```python
from build123d import *

# Parameters (mm, degrees)
F1_DEPTH  = 14
F2_W      = 3
F2_H      = 11.408352
F3_DEPTH  = 18
F5_DEPTH  = 25
F6_R      = 2.8
F7_DEPTH  = 25
F8_R      = 5.75
F9_DEPTH  = 1.5
F10_W     = 3
F10_H     = 9.991856
F11_DEPTH = 18
F13_DEPTH = 25
F14_R     = 2.8
F15_DEPTH = 25
F16_R     = 5.75
F17_DEPTH = 1.5


with BuildPart() as f1:
    # F0 (on Top) → F1 (new body)
    with BuildSketch(Plane.XY):
        with BuildLine():
            Line((-5.879243, 26.052212), (-25.879243, 26.052212))
            Line((-25.879243, 26.052212), (-25.879243, 11.060356))
            ThreePointArc((-25.879243, 11.060356), (-24.293036, 0.175264), (-19.988959, -9.947788))
            ThreePointArc((-19.988959, -9.947788), (-18.281685, -12.624792), (-16.380951, -15.168086))
            ThreePointArc((-16.380951, -15.168086), (-2.161149, -18.102259), (0, -3.744627))
            ThreePointArc((0, -3.744627), (-0.595324, -3.130936), (-1.163612, -2.492127))
            ThreePointArc((-1.163612, -2.492127), (-4.546963, 3.177378), (-5.879243, 9.64386))
            ThreePointArc((-5.879243, 9.64386), (-5.891908, 10.352108), (-5.879243, 11.060356))
            Line((-5.879243, 11.060356), (-5.879243, 26.052212))
        make_face()
        with BuildLine():
            ThreePointArc((-3.681243, -9.899788), (-7.857243, -14.099719), (-12.080969, -9.947788))
            ThreePointArc((-12.080969, -9.947788), (-10.050272, -6.303218), (-5.879243, -6.207635))
            ThreePointArc((-5.879243, -6.207635), (-4.272338, -7.751347), (-3.681243, -9.899788))
        make_face(mode=Mode.SUBTRACT)
        with BuildLine():
            Line((-5.879243, 9.64386), (-5.879243, 11.060356))
            ThreePointArc((-5.879243, 11.060356), (-5.891908, 10.352108), (-5.879243, 9.64386))
        make_face()
        with BuildLine():
            ThreePointArc((0, -3.744627), (-0.554991, -3.093465), (-1.163612, -2.492127))
            ThreePointArc((-1.163612, -2.492127), (-0.595324, -3.130936), (0, -3.744627))
        make_face()
    extrude(amount=F1_DEPTH)

    # F2 (on face) → F3 (join)
    with BuildSketch(Plane.XY.offset(14)):
        Polygon((-5.879243, 26.052212), (-25.879243, 26.052212), (-25.879243, 21.052212), (-22.879243, 21.052212), (-8.879243, 21.052212), (-5.879243, 21.052212), align=None)
        with BuildLine():
            Line((-22.879243, 21.052212), (-25.879243, 21.052212))
            Line((-25.879243, 21.052212), (-25.879243, 11.060356))
            ThreePointArc((-25.879243, 11.060356), (-25.862016, 10.351917), (-25.83308, 9.64386))
            Line((-25.83308, 9.64386), (-22.879243, 9.64386))
            Line((-22.879243, 9.64386), (-22.879243, 21.052212))
        make_face()
        with Locations((-7.379243, 15.348036)):
            Rectangle(F2_W, F2_H)
    extrude(amount=F3_DEPTH)

    # F4 (on face) → F5 (cut)
    with BuildSketch(Plane.YZ.offset(-5.879243)):
        Polygon((9.64386, 14), (23.052212, 32), (9.64386, 32), align=None)
    extrude(amount=-F5_DEPTH, mode=Mode.SUBTRACT)

    # F6 (on face) → F7 (cut)
    with BuildSketch(Plane.XZ.offset(-21.052212)):
        with Locations((-15.879243, 21.657553)):
            Circle(F6_R)
    extrude(amount=-F7_DEPTH, mode=Mode.SUBTRACT)

    # F8 (on face) → F9 (cut)
    with BuildSketch(Plane.XZ.offset(-21.052212)):
        with Locations((-15.879243, 21.657553)):
            Circle(F8_R)
    extrude(amount=-F9_DEPTH, mode=Mode.SUBTRACT)

    # F10 (on face) → F11 (join)
    with BuildSketch(Plane(origin=(0, 0, 0), x_dir=(1, 0, 0), z_dir=(0, 0, -1))):
        with Locations((-24.379243, -16.056284)):
            Rectangle(F10_W, F10_H)
        Polygon((-25.879243, -21.052212), (-25.879243, -26.052212), (-5.879243, -26.052212), (-5.879243, -21.052212), (-8.879243, -21.052212), (-22.879243, -21.052212), align=None)
        with Locations((-7.379243, -16.056284)):
            Rectangle(F10_W, F10_H)
    extrude(amount=F11_DEPTH)

    # F12 (on face) → F13 (cut)
    with BuildSketch(Plane(origin=(-25.879243, 0, 0), x_dir=(0, -1, 0), z_dir=(-1, 0, 0))):
        Polygon((-11.060356, 0), (-22.052212, -18), (-11.060356, -18), align=None)
    extrude(amount=-F13_DEPTH, mode=Mode.SUBTRACT)

    # F14 (on face) → F15 (cut)
    with BuildSketch(Plane.XZ.offset(-21.052212)):
        with Locations((-15.879243, -8.181212)):
            Circle(F14_R)
    extrude(amount=-F15_DEPTH, mode=Mode.SUBTRACT)

    # F16 (on face) → F17 (cut)
    with BuildSketch(Plane.XZ.offset(-21.052212)):
        with Locations((-15.879243, -8.181212)):
            Circle(F16_R)
    extrude(amount=-F17_DEPTH, mode=Mode.SUBTRACT)


solid = f1.part
```
The model under review builds one solid part; all positions refer to its coordinate system, in mm. A direction names the side the tool comes from. Round coordinates to 2 decimals unless told otherwise and drop trailing zeros. Write each loop counter-clockwise with the first axis right and the second up, starting at its lowest first coordinate (ties: lowest second). Pieces come first, ordered by that corner, then holes. Notation, with made-up numbers: (-19.5, 42) - (29.5, 42) arc R32 ccw to (29.5, 78) - close; hole circle Ø1 at (64, 83). An arc over 180 degrees is marked (long way). One line per question, with ' | ' between items.
Item 1: Add section B-B, the plane x = -18. Give the boundary of the cut face in (y, z).
Resolved:
outline: (-13.03, 0) - (21.05, 0) - (21.05, -2.84) - (22.55, -2.84) - (22.55, -6.35) - (26.05, -6.35) - (26.05, 19.83) - (22.55, 19.83) - (22.55, 16.31) - (21.05, 16.31) - (21.05, 14) - (-13.03, 14) - close; (21.05, -16.36) - (22.05, -18) - (26.05, -18) - (26.05, -10.01) - (22.55, -10.01) - (22.55, -13.53) - (21.05, -13.53) - close; (21.05, 27) - (22.55, 27) - (22.55, 23.49) - (26.05, 23.49) - (26.05, 32) - (23.05, 32) - (21.05, 29.32) - close
Item 2: Add section C-C, the plane x = -7.25. Give the boundary of the cut face in (y, z).
Resolved:
outline: (-19.88, 0) - (-14.05, 0) - (-14.05, 14) - (-19.88, 14) - close; (-5.75, 0) - (11.06, 0) - (22.05, -18) - (26.05, -18) - (26.05, 32) - (23.05, 32) - (9.64, 14) - (-5.75, 14) - close
Item 3: For faces 1 (the face through (-5.879, 20, 7)), 2 (the face through (-8.879, 17, -6)), 3 (the face through (-10.568, 21.792, 19.455)), 4 (the face through (-12, 1, 14)), 5 (the face through (-13.21, 24.28, -7.34)), list the 3-axis set-ups (+Z, -Z, +X, -X, +Y, -Y) from which the entire face can be reached by the end or side of a thin tool; tool diameter is ignored.
Resolved:
face 1: +Z, -Z, +X, +Y | face 2: -Z, -Y | face 3: -Y | face 4: +Z, -Y | face 5: +Y, -Y
Item 4: The part is to be moulded in two halves that separate along X. For faces 6 (the face through (-4.513, 3.091, 6.902)), 7 (the face through (-25.879, 20, 7)), 8 (the face through (-2.35, -18.23, 6.9)), 9 (the face through (-13.21, 24.28, 22.5)), say which applies: pulls with the +X half, pulls with the -X half, needs draft (parallel to the pull), parting line crosses it, or undercut.
Resolved:
face 6: pulls with the +X half | face 7: pulls with the -X half | face 8: parting line crosses it | face 9: undercut
Item 5: For P1, Ø4, axis at x = -7, y = -11.5, coming from the +Z side; P2, Ø8, axis at y = 21.5, z = 7, coming from the +X side; P3, Ø8.5, axis at x = -9, y = 8.5, coming from the +Z side; P4, Ø4, axis at x = -15, z = 19, coming from the -Y side, all flat-tipped, find the tip position at first contact; note any pin that passes through.
Resolved:
P1: passes through | P2: stops at x = -5.88 | P3: stops at z = 18.17 | P4: stops at y = 22.55
Item 6: To check wall thickness, follow probe 1 along X at (y, z) = (19, 22.5); probe 2 along X at (y, z) = (15, 7.5); probe 3 along Z at (x, y) = (-19.75, 18.5). State the ranges of each line that lie inside material, in increasing order.
Resolved:
probe 1: x = -25.88 to -22.88, -8.88 to -5.88 | probe 2: x = -25.88 to -5.88 | probe 3: z = 0 to 14
Item 7: Add section A-A, the plane z = 11.5. Give the boundary of the cut face in (x, y), then the cut area to 3 significant figures.
Resolved:
outline: (-25.88, 11.06) arc R42.87 ccw to (-19.99, -9.95) arc R42.87 ccw to (-16.38, -15.17) arc R10 ccw (long way) to (0, -3.74) arc R10 ccw to (-1.16, -2.49) arc R19.81 cw to (-5.88, 9.64) - (-5.88, 26.05) - (-25.88, 26.05) - close; hole (-5.88, -6.21) arc R4.2 ccw (long way) to (-3.68, -9.9) arc R4.2 ccw to start | area: 855 mm2
Item 8: Add section D-D, the plane z = -7. Give the boundary of the cut face in (x, y).
Resolved:
outline: (-25.88, 15.33) - (-22.88, 15.33) - (-22.88, 21.05) - (-21.51, 21.05) - (-21.51, 22.55) - (-18.42, 22.55) - (-18.42, 26.05) - (-25.88, 26.05) - close; (-13.34, 22.55) - (-10.25, 22.55) - (-10.25, 21.05) - (-8.88, 21.05) - (-8.88, 15.33) - (-5.88, 15.33) - (-5.88, 26.05) - (-13.34, 26.05) - close
